```python
from build123d import *

# Parameters (mm, degrees)
BOSS_EXTRUDE1_DEPTH = 124.5
BOSS_EXTRUDE2_DEPTH = 15.5
SKETCH4_W           = 40
SKETCH4_H           = 10
CUT_EXTRUDE3_DEPTH  = 24.5
BOSS_EXTRUDE4_REACH = 155.623
SKETCH8_W           = 50
SKETCH8_H           = 5
SKETCH9_W           = 51
SKETCH9_H           = 5.5
CUT_EXTRUDE4_DEPTH  = 15.5
SKETCH10_R          = 6.75
SKETCH10_R_2        = 1.75
BOSS_EXTRUDE5_DEPTH = 19.4
SKETCH11_R          = 1.75
CUT_EXTRUDE5_DEPTH  = 154.622914957
FILLET1_R           = 10


with BuildPart() as part:
    # Sketch1 → Boss-Extrude1 (new body)
    with BuildSketch(Plane.XY):
        with BuildLine():
            Line((15, -5), (45, -5))
            ThreePointArc((45, -5), (52.071067812, -7.928932188), (55, -15))
            Line((55, -15), (55, -20))
            Line((55, -20), (60, -15))
            Line((60, -15), (60, -10))
            ThreePointArc((60, -10), (57.071067812, -2.928932188), (50, 0))
            Line((50, 0), (10, 0))
            ThreePointArc((10, 0), (2.928932188, -2.928932188), (0, -10))
            Line((0, -10), (0, -15))
            Line((0, -15), (5, -20))
            Line((5, -20), (5, -15))
            ThreePointArc((5, -15), (7.928932188, -7.928932188), (15, -5))
        make_face()
    extrude(amount=BOSS_EXTRUDE1_DEPTH)

    # Sketch2 → Boss-Extrude2 (add)
    with BuildSketch(Plane.XY.offset(124.5)):
        with BuildLine():
            Line((50, 0), (10, 0))
            ThreePointArc((10, 0), (2.928932188, -2.928932188), (0, -10))
            Line((0, -10), (0, -20))
            Line((0, -20), (5, -20))
            Line((5, -20), (55, -20))
            Line((55, -20), (60, -20))
            Line((60, -20), (60, -10))
            ThreePointArc((60, -10), (57.071067812, -2.928932188), (50, 0))
        make_face()
    extrude(amount=BOSS_EXTRUDE2_DEPTH)

    # Sketch4 → Cut-Extrude3 (cut)
    with BuildSketch(Plane.XY.offset(140)):
        with Locations((30, -15)):
            Rectangle(SKETCH4_W, SKETCH4_H)
    extrude(amount=-CUT_EXTRUDE3_DEPTH, mode=Mode.SUBTRACT)

    # Boss-Extrude4: up to this face of the body (flat: up to its plane)
    boss_extrude4_end = Plane(part.part.faces().sort_by_distance((30, -5, 62.25))[0])
    # Sketch8 → Boss-Extrude4 (add, up to the picked face)
    with BuildSketch(Plane.XZ.offset(20), mode=Mode.PRIVATE) as boss_extrude4_sk1:
        with Locations((30, 2.5)):
            Rectangle(SKETCH8_W, SKETCH8_H)
    boss_extrude4_tool1 = split(extrude(boss_extrude4_sk1.sketch, amount=-BOSS_EXTRUDE4_REACH, mode=Mode.PRIVATE), bisect_by=boss_extrude4_end, keep=Keep.BOTH, mode=Mode.PRIVATE)
    add(boss_extrude4_tool1.solids().sort_by(Axis((30, -20, 2.5), (0, 1, 0)))[0])

    # Sketch9 → Cut-Extrude4 (cut)
    with BuildSketch(Plane(origin=(0, -20, 0), x_dir=(-1, 0, 0), z_dir=(0, -1, 0))):
        with Locations((-30, -132.25)):
            Rectangle(SKETCH9_W, SKETCH9_H)
    extrude(amount=-CUT_EXTRUDE4_DEPTH, mode=Mode.SUBTRACT)

    # Sketch10 → Boss-Extrude5 (add)
    with BuildSketch(Plane(origin=(0, 0, 0), x_dir=(1, 0, 0), z_dir=(0, 1, 0))):
        with Locations((20, -11.4)):
            Circle(SKETCH10_R)
        with Locations(Location((20, -11.4, 0), (0, 0, 270))):
            Circle(SKETCH10_R_2, mode=Mode.SUBTRACT)
    boss_extrude5 = extrude(amount=-BOSS_EXTRUDE5_DEPTH)

    # Sketch11 → Cut-Extrude5 (cut, through all)
    with BuildSketch(Plane(origin=(0, 0, 0), x_dir=(1, 0, 0), z_dir=(0, 1, 0))):
        with Locations(Location((20, -11.4, 0), (0, 0, 270))):
            Circle(SKETCH11_R)
    cut_extrude5 = extrude(amount=-CUT_EXTRUDE5_DEPTH, mode=Mode.SUBTRACT)

    # Sketch-Pattern1: Boss-Extrude5, Cut-Extrude5 at 5 more places
    with Locations((20, 0, 0), (20, 0, 79.6), (0, 0, 79.6), (0, 0, 109.6), (20, 0, 109.6)):
        add(boss_extrude5)
        add(cut_extrude5, mode=Mode.SUBTRACT)

    # Fillet1
    # the kernel refuses this fillet: 10 mm, written as the material it takes off along each edge
    with BuildSketch(Plane(origin=(60, -40, 0), x_dir=(0, 0, 1), z_dir=(0, 1, 0)), Plane(origin=(0, -10, 0), x_dir=(0, 0, 1), z_dir=(0, -1, 0))) as fillet1_piece_1:
        with BuildLine():
            CenterArc((FILLET1_R, -FILLET1_R), FILLET1_R, 90, 90)
            Line((0, -FILLET1_R), (0, 0))
            Line((0, 0), (FILLET1_R, 0))
        make_face()
    extrude(amount=30, mode=Mode.SUBTRACT)
    with BuildSketch(Plane(origin=(50, -10, 0), x_dir=(1, 0, 0), z_dir=(0, -1, 0))) as fillet1_piece_2:
        with BuildLine():
            CenterArc((10 - FILLET1_R, FILLET1_R), FILLET1_R, 270, 90)
            Line((10, FILLET1_R), (10, 0))
            Line((10, 0), (10 - FILLET1_R, 0))
        make_face()
    revolve(axis=Axis((50, -10, 0), (0, 0, 1)), revolution_arc=90, mode=Mode.SUBTRACT)
    with BuildSketch(Plane(origin=(10, -10, 0), x_dir=(0, 1, 0), z_dir=(1, 0, 0))) as fillet1_piece_3:
        with BuildLine():
            CenterArc((10 - FILLET1_R, FILLET1_R), FILLET1_R, 270, 90)
            Line((10 - FILLET1_R, 0), (10, 0))
            Line((10, 0), (10, FILLET1_R))
        make_face()
    revolve(axis=Axis((10, -10, 0), (0, 0, 1)), revolution_arc=90, mode=Mode.SUBTRACT)
    with BuildSketch(Plane(origin=(50, 0, 0), x_dir=(0, 0, 1), z_dir=(-1, 0, 0))) as fillet1_piece_4:
        with BuildLine():
            CenterArc((FILLET1_R, -FILLET1_R), FILLET1_R, 90, 90)
            Line((0, -FILLET1_R), (0, 0))
            Line((0, 0), (FILLET1_R, 0))
        make_face()
    extrude(amount=40, mode=Mode.SUBTRACT)


solid = part.part
```
Source: CAD feature listing. Evaluate the final solid. Frame: model axes, mm. A direction names the side the tool comes from. Coordinates: 2 decimals unless noted, no trailing zeros. Loops run counter-clockwise (first coordinate to the right, second up) from the corner with the lowest first, then second, coordinate; pieces in that order, holes last. Notation, with made-up numbers: M 53,-23 L 72,-23 A19 ccw 72,-19 Z; hole C -2,47.5 d10. An arc over 180 degrees is marked long. Use a Markdown table: item, result. Add a question column.
Q1. Section query B-B, the plane x = 31. Return loops of the section in (y, z), and give its area (3 significant figures).
Q2. First-contact query: pin 1 (1.5 mm diameter, centred on y = -17, z = 54, fed in from +X); pin 2 (2.5 mm diameter, centred on x = 39.5, z = 137.5, fed in from -Y); pin 3 (1.5 mm diameter, centred on x = 22, z = 45, fed in from -Y). Flat tips, straight axial feed; report the tip coordinate or a pass-through.
Q3. Section query C-C, the plane z = 39.5. Return loops of the section in (x, y).
Q4. Draft query along X for faces 1 (the cylindrical face through (51.99, -7.85, 63.91)), 2 (the flat face through (0, -13, 74)), 3 (the flat face through (30, 0, 74)). Return one class per face: pulls with the +X half, pulls with the -X half, needs draft (parallel to the pull), parting line crosses it, or undercut.
Q5. Section query A-A, the plane y = -7.5. State how many separate pieces and enclosed holes the cut face has, and give its area (3 significant figures).
Q6. Access query for faces 4 (the cylindrical face through (21.735, -9.564, 90.772)), 5 (the flat face through (50, -15, 127)), 6 (the flat face through (30, -5, 64)). Directions: +Z, -Z, +X, -X, +Y, -Y. A direction counts if a zero-diameter tool reaches every point of the face in a straight line with its end or side. Return the directions, or none.
Q7. Material intervals for L1, parallel to X at y = -14, z = 121; L2, parallel to X at y = -12.5, z = 119; L3, parallel to X at y = -18, z = 90.5, sorted ascending.
Result:
| question | item | result |
|---|---|---|
| 1 | outline | M -20,0 L -10,0 A10 ccw 0,10 L 0,140 L -10,140 L -10,135 L -4.5,135 L -4.5,129.5 L -10,129.5 L -10,124.5 L -5,124.5 L -5,5 L -20,5 Z |
| 1 | area | 801 mm2 |
| 2 | pin 1 | stops at x = 58.75 |
| 2 | pin 2 | stops at y = -10 |
| 2 | pin 3 | stops at y = -5 |
| 3 | outline | M 0,-15 L 5,-20 L 5,-15 A10 cw 15,-5 L 45,-5 A10 cw 55,-15 L 55,-20 L 60,-15 L 60,-10 A10 ccw 50,0 L 10,0 A10 ccw 0,-10 Z |
| 4 | face 1 | undercut |
| 4 | face 2 | pulls with the -X half |
| 4 | face 3 | needs draft |
| 5 | separate pieces | 3 |
| 5 | enclosed holes | 8 |
| 5 | area | 3,550 mm2 |
| 6 | face 4 | +Y, -Y |
| 6 | face 5 | +Z, -Y |
| 6 | face 6 | -Y |
| 7 | L1 | x = 0 to 5.05, 13.25 to 18.25, 21.75 to 26.75, 33.25 to 38.25, 41.75 to 46.75, 54.95 to 60 |
| 7 | L2 | x = 0 to 5.32, 13.55 to 26.45, 33.55 to 46.45, 54.68 to 60 |
| 7 | L3 | x = 3 to 5, 13.27 to 18.32, 21.68 to 26.73, 33.27 to 38.32, 41.68 to 46.73, 55 to 57 |
